Model file for the job. Use its own axes, mm. A direction names the side the tool comes from. Coordinates: 2 decimals unless noted, no trailing zeros. Loops run counter-clockwise (first coordinate to the right, second up) from the corner with the lowest first, then second, coordinate; pieces in that order, holes last. Notation, with made-up numbers: (-8, 21) -> (10, 21) arc R9 ccw to (10, 36) -> close; hole circle Ø2 at (16, -28.75). An arc over 180 degrees is marked (long way). Use one line per item in the form item = value.
```python
from build123d import *

# Parameters (mm, degrees)
F1_DEPTH = 1
F3_DEPTH = 3


with BuildPart() as f1:
    # F0 (on Top) → F1 (new body)
    with BuildSketch(Plane.XY):
        Polygon((-2.187478, 15.077314), (-15, -7.114624), (-12.690599, -7.114624), (-0.455428, 14.077314), (11.779744, -7.114624), (14.089145, -7.114624), (1.276623, 15.077314), align=None)
    extrude(amount=F1_DEPTH)

    # F2 (on face) → F3 (join)
    with BuildSketch(Plane.XY.offset(1)):
        Polygon((-10.223, 1.159382), (-15, -7.114624), (14.089145, -7.114624), (9.312145, 1.159382), align=None)
        Polygon((1.276623, 15.077314), (-2.187478, 15.077314), (-6.271465, 8.003641), (8.305015, 2.903783), align=None)
    extrude(amount=F3_DEPTH)


solid = f1.part
```
Q1. Band-saw the part on A-A, the plane z = 2.4. Write the cut outline in (x, y), and give its area (3 significant figures).
Result:
outline = (-15, -7.11) -> (14.09, -7.11) -> (9.31, 1.16) -> (-10.22, 1.16) -> close; (-6.27, 8) -> (8.31, 2.9) -> (1.28, 15.08) -> (-2.19, 15.08) -> close
area = 284 mm2
Q2. Band-saw the part on B-B, the plane x = 3. Write the cut outline in (y, z).
Result:
outline = (-7.11, 1) -> (1.16, 1) -> (1.16, 4) -> (-7.11, 4) -> close; (4.76, 1) -> (8.09, 1) -> (8.09, 0) -> (12.09, 0) -> (12.09, 4) -> (4.76, 4) -> close
Q3. Band-saw the part on C-C, the plane y = 1.75. Write the cut outline in (x, z), and give its area (3 significant figures).
Result:
outline = (-9.88, 0) -> (-7.57, 0) -> (-7.57, 1) -> (-9.88, 1) -> close; (6.66, 0) -> (8.97, 0) -> (8.97, 1) -> (6.66, 1) -> close
area = 4.62 mm2
Q4. Band-saw the part on D-D, the plane x = -1. Write the cut outline in (y, z).
Result:
outline = (-7.11, 1) -> (1.16, 1) -> (1.16, 4) -> (-7.11, 4) -> close; (6.16, 1) -> (13.13, 1) -> (13.13, 0) -> (15.08, 0) -> (15.08, 4) -> (6.16, 4) -> close
Q5. Which spindle directions (+Z, -Z, +X, -X, +Y, -Y) get a long thin tool onto all of the face, cutting with end or side? Do faces 4 (the face through (7, 2, 1)), 5 (the face through (5.577, 3.63, 0.493)), 6 (the face through (-1, -7.115, 2)). Say none if no direction does.
Result:
face_4 = +Z, -X
face_5 = -Z, -Y
face_6 = +Z, -Z, +X, -X, -Y
Q6. Wall check: line 1 along Y through (x, z) = (-0.25, 1.55); line 2 along Z through (x, y) = (-2.5, -3); line 3 along Y through (x, z) = (1.5, 1.6). Give the ranges that are in metal, low to high.
Result:
line_1 = -7.11 to 1.16, 5.9 to 15.08
line_2 = 1 to 4
line_3 = -7.11 to 1.16, 5.28 to 14.69
Q7. Pin check, flat tips, straight feed: pin 1 Ø0.8 at (x, y) = (8, 2) entering from +Z; pin 2 Ø1 at (x, y) = (-7, 1) entering from -Z; pin 3 Ø2 at (y, z) = (-3, 3) entering from +X. Stop position of each tip, or through.
Result:
pin_1 = 1
pin_2 = 1
pin_3 = 12.29
Q8. Mould opens along Y. For faces 1 (the face through (-6.66, 3.33, 0.49)), 2 (the face through (-1, -3, 1)), 3 (the face through (0, 1.159, 2)) say: released by +Y, released by -Y, zero draft, split by the parting line, or undercut.
Result:
face_1 = released by -Y
face_2 = zero draft
face_3 = undercut
